Read the model definition and answer for the solid it produces. Units are mm, in the model's axes. Face numbers are marked on the shaded views. Round coordinates to 2 decimals unless told otherwise and drop trailing zeros. Order: outer loops, then holes, each group sorted by start corner. A loop starts at its lowest first (then second) coordinate and runs counter-clockwise, first axis right, second up. Notation, with made-up numbers: (64.25, 59) - (78.25, 59) arc R33 ccw to (78.25, 94) - close; hole circle Ø9 at (-29, -1.5). An arc over 180 degrees is marked (long way). Put each result on its own line as item: value. Start each with the question number.
Q1. For a pull along X with two mould halves and no side action, classify the marked faces 1 and 2 as pulls with the +X half, pulls with the -X half, needs draft (parallel to the pull), parting line crosses it, or undercut.
Q2. Find the intervals of material crossed by line 1 along Y through (x, z) = (29.5, -55); line 2 along Y through (x, z) = (13, -26); line 3 along X through (y, z) = (16.5, -54), in increasing order. Write a range as from..to.
Q3. Each of these flat-tipped pins is pushed along its axis until it touches: pin 1 Ø12 at (x, z) = (15.5, -6.5) entering from -Y; pin 2 Ø0.8 at (y, z) = (24, -18.5) entering from +X; pin 3 Ø4 at (x, z) = (40, -27.5) entering from -Y; pin 4 Ø15 at (x, z) = (30, -26) entering from +Y. Where does it stop, or does it pass through?
Q4. Section D-D on y = 17.25 is taken. Give the vertices of the cut face in (x, z).
Q5. Section B-B on x = 47.5 is taken. Give the vertices of the cut face in (y, z).
Q6. Section A-A on y = 5.75 is taken. Give the vertices of the cut face in (x, z).
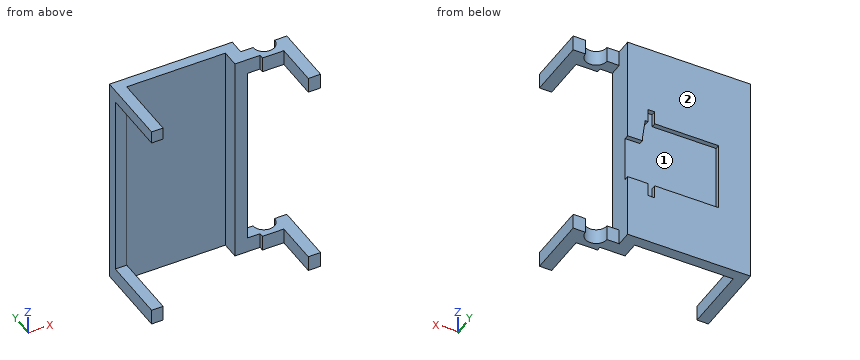
Autodesk Inventor part; units mm, degrees
ref_plane "YZ Plane" through (0, 0, 0) normal (1, 0, 0) x (0, 1, 0)
ref_plane "XZ Plane" through (0, 0, 0) normal (0, 1, 0) x (-1, 0, 0)
ref_plane "XY Plane" through (0, 0, 0) normal (0, 0, 1) x (1, 0, 0)
sketch "Sketch1" plane through (0, 0, 0) normal (0, 1, 0) x (-1, 0, 0)
  line L0 (-40, 0) -> (-40, -60)
  line L1 (0, -60) -> (0, 0)
  line L2 (-40, -60) -> (-55, -60)
  line L3 (-55, -60) -> (-55, -65)
  line L4 (-55, -65) -> (0, -65)
  line L5 (0, -65) -> (0, -60)
  line L6 (-40, 0) -> (-55, 0)
  line L7 (-55, 0) -> (-55, 5)
  line L8 (-55, 5) -> (0, 5)
  line L9 (0, 5) -> (0, 0)
extrude "Extrusion1" add sketch "Sketch1" along normal blind 25
sketch "Sketch2" plane through (0, 25, 0) normal (0, 1, 0) x (1, 0, 0)
  line L0 (55, 0) -> (40, 0)
  line L1 (40, 0) -> (55, 0)
  line L2 (55, 0) -> (55, -5)
  line L3 (55, -5) -> (40, -5)
  line L4 (40, -5) -> (40, 0)
  line L5 (40, 0) -> (40, 60)
  line L6 (55, 60) -> (55, 65)
  line L7 (40, 60) -> (55, 60)
  line L8 (55, 60) -> (55, 65)
  line L9 (55, 65) -> (40, 65)
  line L10 (40, 65) -> (40, 60)
  point P0 (0, 0)
extrude "Extrusion2" cut sketch "Sketch2" against normal blind 5
sketch "Sketch3" plane through (0, 0, 5) normal (0, 0, 1) x (1, 0, 0)
  line L0 (55, 20) -> (40, 20)
  circle A0 centre (47.5, 20) radius 3.5
  point P0 (0, 0)
  dimension "d10" = 7
extrude "Extrusion3" cut sketch "Sketch3" against normal through all
sketch "Sketch4" plane through (0, 25, 0) normal (0, 1, 0) x (1, 0, 0)
  line L0 (40, 0) -> (40, 60)
  line L1 (40, 44.0004) -> (40, 29.1004)
  line L2 (31.2, 48.3504) -> (31.2, 44.0004)
  line L3 (31.2, 44.0004) -> (10.4, 44.0004)
  line L4 (10.4, 44.0004) -> (10.4, 21.4004)
  line L5 (10.4, 21.4004) -> (31.2, 21.4004)
  line L6 (31.2, 21.4004) -> (31.2, 17.0504)
  line L7 (31.2, 17.0504) -> (33.35, 17.0504)
  line L8 (33.35, 17.0504) -> (33.35, 21.4004)
  line L9 (31.2, 48.3504) -> (33.35, 48.3504)
  line L10 (33.35, 48.3504) -> (33.35, 44.0004)
  line L11 (33.35, 44.0004) -> (40, 44.0004)
  line L12 (40, 29.1004) -> (35.1995, 29.1004)
  line L13 (35.1995, 29.1004) -> (35.1995, 28.1004)
  line L14 (33.35, 21.4004) -> (34.3, 21.4004)
  line L15 (34.3, 21.4004) -> (35.1995, 28.1004)
  point P0 (0, 0)
  dimension "d13" = 14.9
  dimension "d19" = 20.8
  dimension "d20" = 22.6
  dimension "d21" = 20.8
  dimension "d32" = 2.15
  dimension "d33" = 2.15
  dimension "d34" = 1
  dimension "d35" = 0.95
extrude "Extrusion4" cut sketch "Sketch4" against normal blind 1.5
sketch "Sketch5" plane through (0, 0, 5) normal (0, 0, 1) x (1, 0, 0)
  line L0 (55, 0) -> (0, 0)
  line L1 (44.0382, 15.8995) -> (35.8479, 15.8995)
  line L2 (3.7342, 15.8995) -> (3.7342, 0)
  line L3 (3.7342, 0) -> (51, 0)
  line L4 (51, 0) -> (51, 14.5037)
  line L5 (51, 14.5037) -> (44.0382, 14.5037)
  line L6 (44.0382, 14.5037) -> (44.0382, 15.8995)
  line L7 (3.7342, 15.8995) -> (3.7342, 21.5553)
  line L8 (3.7342, 21.5553) -> (35.8479, 21.5553)
  line L9 (35.8479, 21.5553) -> (35.8479, 15.8995)
extrude "Extrusion5" cut sketch "Sketch5" against normal through all
sketch "Sketch9" plane through (0, 0, -65) normal (-1, 0, 0) x (0, 0, 1)
  line L0 (70, 0) -> (65, 0)
  line L1 (5.02, 21.545) -> (65.98, 21.545)
  line L2 (65.98, 21.545) -> (65.98, 0)
  line L3 (65.98, 0) -> (5.02, 0)
  line L4 (5.02, 0) -> (5.02, 21.545)
  dimension "d29" = 60.96
extrude "Extrusion6" cut sketch "Sketch9" against normal blind 10
properties part number "servo_sandboxv3"
Findings:
1. face 1: undercut
1. face 2: needs draft
2. line 1: 21.56..25
2. line 2: 21.56..23.5
2. line 3: 35.85..40
3. pin 1: y = 21.56
3. pin 2: x = 40
3. pin 3: y = 15.9
3. pin 4: y = 25
4. outline: (0, -65) - (3.73, -65) - (3.73, -59.98) - (0, -59.98) - close; (0, 0.98) - (3.73, 0.98) - (3.73, 5) - (0, 5) - close; (35.85, -65) - (45.33, -65) - (45.33, -60) - (40, -60) - (40, 0) - (45.33, 0) - (45.33, 5) - (35.85, 5) - close; (49.67, -65) - (55, -65) - (55, -60) - (49.67, -60) - close; (49.67, 0) - (55, 0) - (55, 5) - (49.67, 5) - close
5. outline: (14.5, -65) - (16.5, -65) - (16.5, -60) - (14.5, -60) - close; (14.5, 0) - (16.5, 0) - (16.5, 5) - (14.5, 5) - close
6. outline: (0, -65) - (3.73, -65) - (3.73, -59.98) - (0, -59.98) - close; (0, 0.98) - (3.73, 0.98) - (3.73, 5) - (0, 5) - close; (51, -65) - (55, -65) - (55, -60) - (51, -60) - close; (51, 0) - (55, 0) - (55, 5) - (51, 5) - close
